```python
from build123d import *

# Parameters (mm, degrees)
CROQUIS3_R            = 1.25
CORTAR_EXTRUIR1_DEPTH = 5


with BuildPart() as part:
    # Croquis2 → Revolución1 (revolve)
    with BuildSketch(Plane.XY):
        Polygon((0, 19), (-1.5, 19), (-1.5, 3.734066961), (-4.5, 3.734066961), (-4.5, 1.654780276), (-9, 1.654780276), (-13.5, -2.31384669), (-13.5, -14), (-12.264104671, -19), (0, -19), align=None)
    revolve(axis=Axis((0, -19, 0), (0, 1, 0)))

    # Croquis3 → Cortar-Extruir1 (cut, symmetric)
    with BuildSketch(Plane(origin=(0, -19, 0), x_dir=(1, 0, 0), z_dir=(0, 1, 0))):
        with Locations((-9, 0)):
            Circle(CROQUIS3_R)
        with Locations((9, 0)):
            Circle(CROQUIS3_R)
        with Locations((0, -7)):
            Circle(CROQUIS3_R)
        with Locations((0, 7)):
            Circle(CROQUIS3_R)
    extrude(amount=CORTAR_EXTRUIR1_DEPTH, both=True, mode=Mode.SUBTRACT)


solid = part.part
```
Check sheet for the modelled part. Datum: model origin and axes. Units: mm. A direction names the side the tool comes from. Coordinates: 2 decimals unless noted, no trailing zeros. Order: outer loops, then holes, each group sorted by start corner. A loop starts at its lowest first (then second) coordinate and runs counter-clockwise, first axis right, second up. Notation, with made-up numbers: M 52.25,22 L 56.25,22 A20 cw 56.25,39 Z; hole C 12.25,54.5 d7. An arc over 180 degrees is marked long. Write each question's results on one line, items separated by ' | '. Start each with the question number.
1. Material ranges on probe 1 along X at (y, z) = (-15, 0); probe 2 along Y at (x, z) = (2, -4.5); probe 3 along X at (y, z) = (-16.75, 7), recorded low to high.
2. Cross-section at D-D on y = -13. Record the cut outline in (x, z).
3. Cross-section at B-B on x = 0. Record the cut outline in (y, z).
4. Cross-section at A-A on z = 0. Record the cut outline in (x, y).
5. Access from +Z, -Z, +X, -X, +Y, -Y to the whole of each face (thin tool, end or side, straight path). Record for faces 4 (the face through (9, -14, 0)), 5 (the face through (0.59, 2.68, 4.46)), 6 (the face through (0, -19, 0)).
6. Go/stop test with flat-tipped pins: P1, Ø2, axis at x = -4.5, y = 3.5, coming from the +Z side; P2, Ø5, axis at y = 4, z = 5, coming from the -X side; P3, Ø3, axis at x = -8.5, z = -4.5, coming from the +Y side. Record where each tip stops, or that it passes through.
7. Cross-section at C-C on y = 4.5. Record the cut outline in (x, z), and give its area (3 significant figures).
8. Mould release check, pull along Z, two halves, no side actions. Record for faces 1 (the face through (1.5, 11.26, 0.07)), 2 (the face through (4, 1.655, -4)), 3 (the face through (0, -14, -7)): +Z half, -Z half, draft (parallel to the pull), parting line (faces both ways), or undercut.
Checks:
1) probe 1: x = -13.25 to -10.25, -7.75 to 7.75, 10.25 to 13.25 | probe 2: y = -19 to 1.65 | probe 3: x = -10.74 to -1.25, 1.25 to 10.74
2) outline: C 0,0 d27
3) outline: M -19,-12.26 L -14,-13.5 L -2.31,-13.5 L 1.65,-9 L 1.65,-4.5 L 3.73,-4.5 L 3.73,-1.5 L 19,-1.5 L 19,1.5 L 3.73,1.5 L 3.73,4.5 L 1.65,4.5 L 1.65,9 L -2.31,13.5 L -14,13.5 L -19,12.26 L -19,8.25 L -14,8.25 L -14,5.75 L -19,5.75 L -19,-5.75 L -14,-5.75 L -14,-8.25 L -19,-8.25 Z
4) outline: M -13.5,-14 L -12.26,-19 L -10.25,-19 L -10.25,-14 L -7.75,-14 L -7.75,-19 L 7.75,-19 L 7.75,-14 L 10.25,-14 L 10.25,-19 L 12.26,-19 L 13.5,-14 L 13.5,-2.31 L 9,1.65 L 4.5,1.65 L 4.5,3.73 L 1.5,3.73 L 1.5,19 L -1.5,19 L -1.5,3.73 L -4.5,3.73 L -4.5,1.65 L -9,1.65 L -13.5,-2.31 Z
5) face 4: -Y | face 5: +Y | face 6: +Z, -Z, +X, -X, -Y
6) P1: stops at z = 2.83 | P2: stops at x = -7.99 | P3: stops at y = 1.65
7) outline: C 0,0 d3 | area: 7.07 mm²
8) face 1: parting line | face 2: draft | face 3: undercut
